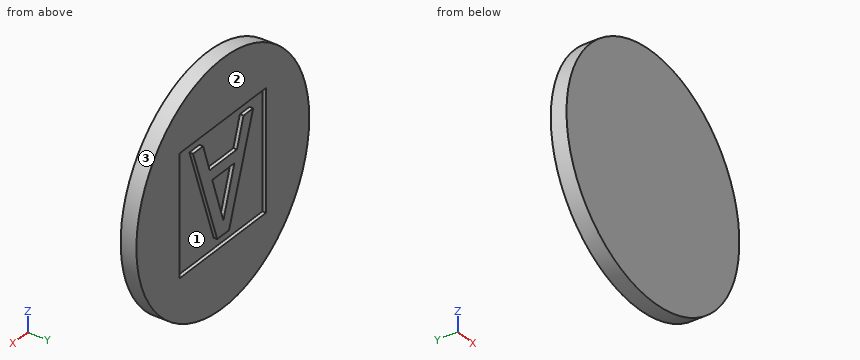
Autodesk Inventor part; units mm, degrees
ref_plane "YZ Plane" through (0, 0, 0) normal (1, 0, 0) x (0, 1, 0)
ref_plane "XZ Plane" through (0, 0, 0) normal (0, 1, 0) x (-1, 0, 0)
ref_plane "XY Plane" through (0, 0, 0) normal (0, 0, 1) x (1, 0, 0)
sketch "Sketch1" plane through (0, 0, 0) normal (0, 1, 0) x (-1, 0, 0)
  circle A0 centre (0, 0) radius 20
  dimension "d0" = 40
extrude "Extrusion1" add sketch "Sketch1" along normal blind 2.6
sketch "Sketch2" plane through (0, 2.6, 0) normal (0, 1, 0) x (1, 0, 0)
  line L0 (-10, -10) -> (-10, 10)
  line L1 (-10, 10) -> (10, 10)
  line L2 (10, 10) -> (10, -10)
  line L3 (10, -10) -> (-10, -10)
  line L4 (-10, -10) -> (10, 10) construction
  line L5 (-10, 10) -> (10, -10) construction
  point P0 (0, 0)
  dimension "d3" = 20
  dimension "d4" = 20
extrude "Extrusion2" cut sketch "Sketch2" against normal blind 0.6
sketch "Sketch3" plane through (0, 2, 0) normal (0, 1, 0) x (1, 0, 0)
  line L0 (-6.9184, 8.3) -> (6.9911, 8.3) construction
  line L1 (6.9911, 8.3) -> (6.9911, -8.3) construction
  line L2 (6.9911, -8.3) -> (-6.9184, -8.3) construction
  line L3 (-6.9184, -8.3) -> (-6.9184, 8.3) construction
  line L4 (-7.026, -8.3) -> (-1.4299, 8.3)
  line L5 (-1.4299, 8.3) -> (1.2874, 8.3)
  line L6 (1.2874, 8.3) -> (6.8835, -8.3)
  line L7 (6.8835, -8.3) -> (4.5563, -8.3)
  line L8 (4.5563, -8.3) -> (3.0496, -3.659)
  line L9 (3.0496, -3.659) -> (-3.2863, -3.659)
  line L10 (-3.2863, -3.659) -> (-4.793, -8.3)
  line L11 (-4.793, -8.3) -> (-7.026, -8.3)
  line L12 (2.4443, -1.7757) -> (-0.1251, 6.04)
  line L13 (-0.1251, 6.04) -> (-2.681, -1.7757)
  line L14 (-2.681, -1.7757) -> (2.4443, -1.7757)
  point P0 (0, 0)
extrude "Extrusion3" add sketch "Sketch3" along normal blind 0.6
properties part number "TopMarkerPreset"
Design review of the part built by this model. Coordinates are the model's own, in mm. Face numbers are marked on the shaded views. Give positions to 0.01 mm unless a question says otherwise; leave off trailing zeros. Write each loop counter-clockwise with the first axis right and the second up, starting at its lowest first coordinate (ties: lowest second). Pieces come first, ordered by that corner, then holes.
(1) Add section A-A (z = -2). Give the boundary of the cut face in (x, y).
Checked values:
outline: (-19.9, 0) - (19.9, 0) - (19.9, 2.6) - (10, 2.6) - (10, 2) - (3.41, 2) - (3.41, 2.6) - (1.2, 2.6) - (1.2, 2) - (-1.45, 2) - (-1.45, 2.6) - (-3.55, 2.6) - (-3.55, 2) - (-10, 2) - (-10, 2.6) - (-19.9, 2.6) - close
(2) Clearance check with flat-ended pins moving along their axes: pin 1 Ø0.5 at (y, z) = (2.5, 4.5) entering from +X; pin 2 Ø0.7 at (y, z) = (2, 4) entering from -X; pin 3 Ø0.5 at (x, y) = (1, 2.5) entering from -Z. State where each tip first meets the part, or that it passes through.
Checked values:
pin 1: stops at x = 19.54
pin 2: stops at x = -19.66
pin 3: stops at z = -19.99
(3) Add section D-D (x = 13). Give the boundary of the cut face in (y, z).
Checked values:
outline: (0, -15.2) - (2.6, -15.2) - (2.6, 15.2) - (0, 15.2) - close
(4) Add section C-C (z = 10.5). Give the boundary of the cut face in (x, y), and give its area (3 significant figures).
Checked values:
outline: (-17.02, 0) - (17.02, 0) - (17.02, 2.6) - (-17.02, 2.6) - close
area: 88.5 mm2
(5) Wall thickness on line 1 along Y through (x, z) = (-0.5, 0); line 2 along X through (y, z) = (2.25, -4); line 3 along X through (y, z) = (1.5, 17): over which ranges is each line inside the solid? List them lowest first.
Checked values:
line 1: y = 0 to 2
line 2: x = -19.6 to -10, -2.88 to -0.79, 0.55 to 2.74, 10 to 19.6
line 3: x = -10.54 to 10.54
(6) Add section B-B (x = 8.5). Give the boundary of the cut face in (y, z).
Checked values:
outline: (0, -18.1) - (2.6, -18.1) - (2.6, -10) - (2, -10) - (2, 10) - (2.6, 10) - (2.6, 18.1) - (0, 18.1) - close
(7) Mouldability with a two-part tool opening along X and no side actions: class the marked faces 1, 2 and 3 as +X half, -X half, draft (parallel to the pull), parting line (faces both ways), or undercut.
Checked values:
face 1: undercut
face 2: draft
face 3: parting line
